```python
from build123d import *

# Parameters (mm, degrees)
SKETCH1_R                                         = 44.5
BOSS_EXTRUDE1_DEPTH                               = 3
SKETCH2_R                                         = 29.5
CUT_EXTRUDE1_DEPTH                                = 3
CSK_FOR_0_FLAT_HEAD_MACHINE_SCREW_100_D           = 1.778
CSK_FOR_0_FLAT_HEAD_MACHINE_SCREW_100_CSINK_D     = 3.0226
CSK_FOR_0_FLAT_HEAD_MACHINE_SCREW_100_CSINK_ANGLE = 100
CIRPATTERN1_COUNT                                 = 8


with BuildPart() as part:
    # Sketch1 → Boss-Extrude1 (new body)
    with BuildSketch(Plane.XY):
        Circle(SKETCH1_R)
    extrude(amount=BOSS_EXTRUDE1_DEPTH)

    # Sketch2 → Cut-Extrude1 (cut)
    with BuildSketch(Plane.XY.offset(3)):
        Circle(SKETCH2_R)
    extrude(amount=-CUT_EXTRUDE1_DEPTH, mode=Mode.SUBTRACT)

    # CSK for #0 Flat Head Machine Screw (100)1 (through all)
    with Locations(Plane.XY.offset(3)):
        with Locations((0, 42)):
            csk_for_0_flat_head_machine_screw_100 = CounterSinkHole(CSK_FOR_0_FLAT_HEAD_MACHINE_SCREW_100_D / 2, CSK_FOR_0_FLAT_HEAD_MACHINE_SCREW_100_CSINK_D / 2, counter_sink_angle=CSK_FOR_0_FLAT_HEAD_MACHINE_SCREW_100_CSINK_ANGLE)

    # CirPattern1: CSK for #0 Flat Head Machine Screw (100)1 ×8 about axis
    cirpattern1_axis = Axis((0, 0, 0), (0, 0, 1))
    for i in range(1, CIRPATTERN1_COUNT):
        add(csk_for_0_flat_head_machine_screw_100.rotate(cirpattern1_axis, i * 360 / CIRPATTERN1_COUNT), mode=Mode.SUBTRACT)


solid = part.part
```
The listing builds one solid part. Answer for the finished solid, in the listing's coordinates (mm). Coordinates: 2 decimals unless noted, no trailing zeros. Loops run counter-clockwise (first coordinate to the right, second up) from the corner with the lowest first, then second, coordinate; pieces in that order, holes last. Notation, with made-up numbers: (73, 28) -> (120, 28) arc R25 cw to (120, 58) -> close; hole circle Ø6 at (86.5, -31). An arc over 180 degrees is marked (long way). Return JSON: item names as keys, results as strings. Group by question number.
(1) Determine the mould class of faces 1 (the cylindrical face through (28.14, 8.86, 1.52)), 2 (the flat face through (29, -9, 0)), 3 (the cylindrical face through (-32.798, 30.075, 1.479)) for opening direction Y: released by +Y, released by -Y, zero draft, split by the parting line, or undercut.
(2) A cutting plane is placed at B-B on y = -4.5. Write down the section's boundary in (x, z), and give its area (3 significant figures).
(3) Given pin 1 Ø1.6 at (x, y) = (-29.7, -29.7) entering from +Z; pin 2 Ø2 at (x, y) = (-42, 0) entering from +Z; pin 3 Ø2.5 at (x, y) = (0, -42) entering from +Z, each flat-ended and moving along its own axis, determine where each tip first touches the part or whether it passes through.
(4) A cutting plane is placed at D-D on x = 35. Write down the section's boundary in (y, z), and give its area (3 significant figures).
(5) A cutting plane is placed at C-C on z = 0.95. Count the separate pieces of the cut face and the enclosed holes in it, and give its area (3 significant figures).
(6) A cutting plane is placed at A-A on x = -18. Write down the section's boundary in (y, z), and give its area (3 significant figures).
(7) Find the intervals of material crossed by probe 1 along Y at (x, z) = (0, 1.5); probe 2 along X at (y, z) = (1, 2.3); probe 3 along X at (y, z) = (20.5, 2.25), in increasing order. Write a range as from..to.
The answers:
{
 "1": {"face 1": "undercut", "face 2": "zero draft", "face 3": "split by the parting line"},
 "2": {"outline": "(-44.27, 0) -> (-29.15, 0) -> (-29.15, 3) -> (-44.27, 3) -> close; (29.15, 0) -> (44.27, 0) -> (44.27, 3) -> (29.15, 3) -> close", "area": "90.7 mm^2"},
 "3": {"pin 1": "passes through", "pin 2": "stops at z = 2.57", "pin 3": "stops at z = 2.78"},
 "4": {"outline": "(-27.48, 0) -> (27.48, 0) -> (27.48, 3) -> (-27.48, 3) -> close", "area": "165 mm^2"},
 "5": {"separate pieces": "1", "enclosed holes": "9", "area": "3,470 mm^2"},
 "6": {"outline": "(-40.7, 0) -> (-23.37, 0) -> (-23.37, 3) -> (-40.7, 3) -> close; (23.37, 0) -> (40.7, 0) -> (40.7, 3) -> (23.37, 3) -> close", "area": "104 mm^2"},
 "7": {"probe 1": "y = -44.5..-42.89, -41.11..-29.5, 29.5..41.11, 42.89..44.5", "probe 2": "x = -44.49..-29.48, 29.48..44.49", "probe 3": "x = -39.5..-21.21, 21.21..39.5"}
}
